```python
from build123d import *

# Parameters (mm, degrees)
SKETCH1_R           = 19.25
SKETCH1_R_2         = 4
BOSS_EXTRUDE1_DEPTH = 4
SKETCH1_4_R         = 4
BOSS_EXTRUDE2_DEPTH = 27.15
CUT_EXTRUDE1_START  = -1.932
SKETCH6_R           = 4
SKETCH6_R_2         = 3.356
CUT_EXTRUDE1_DEPTH  = 1.932
SKETCH7_R           = 2.25
CUT_EXTRUDE2_DEPTH  = 36.735801376
SKETCH8_R           = 2.5
CUT_EXTRUDE3_DEPTH  = 5
CHAMFER1_SIZE       = 2
CHAMFER1_SIZE2      = 0.727940469
SKETCH9_W           = 0.25
SKETCH9_H           = 2.75
CHAMFER3_SIZE       = 0.3
CHAMFER3_SIZE_2     = 0.210062261


with BuildPart() as part:
    # Sketch1 → Boss-Extrude1 (new body)
    # profile 1 of 2: a face of its own
    with BuildSketch(Plane(origin=(0, 0, 0), x_dir=(1, 0, 0), z_dir=(0, 1, 0))):
        with Locations(Location((0, 0, 0), (0, 0, 270))):
            Circle(SKETCH1_R)
        with BuildLine():
            ThreePointArc((2, -16.5), (0, -18.5), (-2, -16.5))
            Line((-2, -16.5), (-2, -16.378339354))
            ThreePointArc((-2, -16.378339354), (-14.289419162, -8.25), (-15.184057953, 6.45711887))
            Line((-15.184057953, 6.45711887), (-15.289419162, 6.517949192))
            ThreePointArc((-15.289419162, 6.517949192), (-16.02146997, 9.25), (-13.289419162, 9.982050808))
            Line((-13.289419162, 9.982050808), (-13.184057953, 9.921220485))
            ThreePointArc((-13.184057953, 9.921220485), (0, 16.5), (13.184057953, 9.921220485))
            Line((13.184057953, 9.921220485), (13.289419162, 9.982050808))
            ThreePointArc((13.289419162, 9.982050808), (16.02146997, 9.25), (15.289419162, 6.517949192))
            Line((15.289419162, 6.517949192), (15.184057953, 6.45711887))
            ThreePointArc((15.184057953, 6.45711887), (16.167667677, 3.294923655), (16.5, 0))
            ThreePointArc((16.5, 0), (12.354149101, -10.937321427), (2, -16.378339354))
            Line((2, -16.378339354), (2, -16.5))
        make_face(mode=Mode.SUBTRACT)
    # profile 2 of 2: a face of its own
    with BuildSketch(Plane(origin=(0, 0, 0), x_dir=(1, 0, 0), z_dir=(0, 1, 0))):
        with BuildLine():
            ThreePointArc((-15.184057953, 6.45711887), (-14.289419162, -8.25), (-2, -16.378339354))
            Line((-2, -16.378339354), (-2, -13.96))
            ThreePointArc((-2, -13.96), (0, -11.96), (2, -13.96))
            Line((2, -13.96), (2, -16.378339354))
            ThreePointArc((2, -16.378339354), (12.354149101, -10.937321427), (16.5, 0))
            ThreePointArc((16.5, 0), (16.167667677, 3.294923655), (15.184057953, 6.45711887))
            Line((15.184057953, 6.45711887), (13.089714637, 5.247949192))
            ThreePointArc((13.089714637, 5.247949192), (10.357663829, 5.98), (11.089714637, 8.712050808))
            Line((11.089714637, 8.712050808), (13.184057953, 9.921220485))
            ThreePointArc((13.184057953, 9.921220485), (0, 16.5), (-13.184057953, 9.921220485))
            Line((-13.184057953, 9.921220485), (-11.094979939, 8.715090731))
            Line((-11.094979939, 8.715090731), (-11.089714637, 8.712050808))
            ThreePointArc((-11.089714637, 8.712050808), (-10.357663829, 5.98), (-13.089714637, 5.247949192))
            Line((-13.089714637, 5.247949192), (-15.184057953, 6.45711887))
        make_face()
        with Locations(Location((0, 0, 0), (0, 0, 270))):
            Circle(SKETCH1_R_2, mode=Mode.SUBTRACT)
    extrude(amount=-BOSS_EXTRUDE1_DEPTH)

    # Sketch1<4> → Boss-Extrude2 (add)
    with BuildSketch(Plane(origin=(0, 0, 0), x_dir=(1, 0, 0), z_dir=(0, 1, 0))):
        with Locations(Location((0, 0, 0), (0, 0, 270))):
            Circle(SKETCH1_4_R)
    extrude(amount=-BOSS_EXTRUDE2_DEPTH)

    # Sketch2 → Cut-Revolve4 (revolve, cut)
    with BuildSketch(Plane(origin=(0, 0, 0), x_dir=(0, 0, -1), z_dir=(1, 0, 0)), mode=Mode.PRIVATE) as cut_revolve4_sk:
        Polygon((0, -27.15), (0.8, -27.15), (0.8, -25.15), (1, 0), (0, 0), align=None)
    revolve(cut_revolve4_sk.sketch.rotate(Axis((0, 0, 0), (0, -1, 0)), 180), axis=Axis((0, 0, 0), (0, -1, 0)), mode=Mode.SUBTRACT)

    # Sketch5 → Cut-Revolve8 (revolve, cut)
    with BuildSketch(Plane.XY, mode=Mode.PRIVATE) as cut_revolve8_sk:
        Polygon((0, -7), (-2.55, -5.527756814), (-2.55, 0), (0, 0), align=None)
    revolve(cut_revolve8_sk.sketch.rotate(Axis((0, 0, 0), (0, -1, 0)), 270), axis=Axis((0, 0, 0), (0, -1, 0)), mode=Mode.SUBTRACT)

    # Sketch6 → Cut-Extrude1 (cut)
    with BuildSketch(Plane.XZ.offset(27.15).offset(CUT_EXTRUDE1_START)):
        with Locations(Location((0, 0, 0), (0, 0, 90))):
            Circle(SKETCH6_R)
        with Locations(Location((0, 0, 0), (0, 0, 270))):
            Circle(SKETCH6_R_2, mode=Mode.SUBTRACT)
    extrude(amount=CUT_EXTRUDE1_DEPTH, mode=Mode.SUBTRACT)

    # Sketch7 → Cut-Extrude2 (cut, through all)
    with BuildSketch(Plane.XZ.offset(4)):
        with Locations(Location((0, -6.25, 0), (0, 0, 270))):
            Circle(SKETCH7_R)
    extrude(amount=-CUT_EXTRUDE2_DEPTH, mode=Mode.SUBTRACT)

    # Sketch8 → Cut-Extrude3 (cut)
    with BuildSketch(Plane(origin=(0, -23, 0), x_dir=(1, 0, 0), z_dir=(0, 1, 0))):
        with Locations((0, 4)):
            Circle(SKETCH8_R)
    extrude(amount=CUT_EXTRUDE3_DEPTH, mode=Mode.SUBTRACT)

    # Chamfer1
    chamfer1_edges = [part.edges().sort_by_distance(p)[0] for p in [
        (0, -18, -4),
    ]]
    chamfer1_side = [part.faces().sort_by_distance(p)[0] for p in [
        (0, -14.609, -4),
    ]]
    chamfer(chamfer1_edges, length=CHAMFER1_SIZE, length2=CHAMFER1_SIZE2, reference=chamfer1_side[0])

    # Sketch9 → Cut-Revolve9 (revolve, cut)
    with BuildSketch(Plane(origin=(0, 0, 0), x_dir=(0, 0, -1), z_dir=(1, 0, 0)), mode=Mode.PRIVATE) as cut_revolve9_sk:
        with Locations((-3.875, -20.5)):
            Rectangle(SKETCH9_W, SKETCH9_H)
    revolve(cut_revolve9_sk.sketch.rotate(Axis((0, -27.15, 0), (0, 1, 0)), 143.580086271), axis=Axis((0, -27.15, 0), (0, 1, 0)), mode=Mode.SUBTRACT)

    # Chamfer3
    # the kernel refuses this chamfer: 0.3, 0.210062261 mm, written as the material it takes off along each edge
    with BuildSketch(Plane(origin=(0, -21.875, 0), x_dir=(-0.42752924874280274, 0, -0.9040015162981834), z_dir=(0.9040015162981834, 0, -0.42752924874280274))) as chamfer3_piece_1_section:
        Polygon((4 - CHAMFER3_SIZE, 0), (4, -CHAMFER3_SIZE_2 * 1.0000000022), (4, 0), align=None)
    chamfer3_piece_1 = revolve(axis=Axis((0, -21.875, 0), (0, 1, 0)), revolution_arc=154.689138052, mode=Mode.PRIVATE)
    chamfer3_piece_1 = chamfer3_piece_1 - Plane(origin=(0, -21.995167344, 0), x_dir=(0.593698599754949, 0, -0.8046874999955033), z_dir=(0, -1, 0)) * Cylinder(3.75, 16, mode=Mode.PRIVATE)
    add(chamfer3_piece_1, mode=Mode.SUBTRACT)
    with BuildSketch(Plane(origin=(0, -21.875, 0), x_dir=(0, 0, 1), z_dir=(-1, 0, 0))) as chamfer3_piece_2_section:
        Polygon((4 - CHAMFER3_SIZE, 0), (4, -CHAMFER3_SIZE_2 * 1.0000000022), (4, 0), align=None)
    chamfer3_piece_2 = revolve(axis=Axis((0, -21.875, 0), (0, 1, 0)), revolution_arc=154.689138052, mode=Mode.PRIVATE)
    chamfer3_piece_2 = chamfer3_piece_2 - Plane(origin=(0, -21.995167344, 0), x_dir=(0.593698599754949, 0, -0.8046874999955033), z_dir=(0, -1, 0)) * Cylinder(3.75, 16, mode=Mode.PRIVATE)
    add(chamfer3_piece_2, mode=Mode.SUBTRACT)


solid = part.part
```
The model under review builds one solid part; all positions refer to its coordinate system, in mm. A direction names the side the tool comes from. Round coordinates to 2 decimals unless told otherwise and drop trailing zeros. Order: outer loops, then holes, each group sorted by start corner. A loop starts at its lowest first (then second) coordinate and runs counter-clockwise, first axis right, second up.
(1) Take a section at C-C, the plane z = 8.5. State the section outline as (x, y) points, plus the area to 3 significant figures.
Working result:
outline: (-17.27, -4) - (17.27, -4) - (17.27, 0) - (-17.27, 0) - close
area: 138 mm2
(2) Take a section at B-B, the plane y = -10.25. State the section outline as (x, z) points, plus the area to 3 significant figures.
Working result:
outline: circle Ø8 at (0, 0); hole circle Ø1.84 at (0, 0)
area: 47.6 mm2
(3) Take a section at D-D, the plane x = -7. State the section outline as (y, z) points, plus the area to 3 significant figures.
Working result:
outline: (-4, -17.93) - (0, -17.93) - (0, 17.93) - (-4, 17.93) - close
area: 143 mm2
(4) Tool access review of faces 4 (the face through (0, -18, -2)), 5 (the face through (-1.532, -23.63, 3.695)), 6 (the face through (-2, -2, 15)), 7 (the face through (-0.77, -2.73, 2.43)): name each direction out of +Z, -Z, +X, -X, +Y, -Y from which nothing blocks a thin tool from reaching the whole face with its end or side.
Working result:
face 4: -Z
face 5: -Y
face 6: +Y, -Y
face 7: +Y
(5) Take a section at A-A, the plane y = -2. State the section outline as (x, z) points.
Working result:
outline: circle Ø38.5 at (0, 0); hole (-15.29, -6.52) arc R2 ccw to (-13.29, -9.98) - (-11.09, -8.71) arc R2 ccw to (-13.09, -5.25) - close; hole circle Ø5.1 at (0, 0); hole circle Ø4.5 at (0, -6.25); hole (-2, 13.96) arc R2 ccw to (2, 13.96) - (2, 16.5) arc R2 ccw to (-2, 16.5) - close; hole (11.09, -8.71) - (13.29, -9.98) arc R2 ccw to (15.29, -6.52) - (13.09, -5.25) arc R2 ccw to start
(6) For P1, Ø5, axis at x = -8, z = 6, coming from the +Y side; P2, Ø1.5, axis at y = -16, z = 4, coming from the -X side; P3, Ø3, axis at x = 0, z = 0, coming from the +Y side; P4, Ø5, axis at x = -3, z = -5.5, coming from the -Y side, all flat-tipped, find the tip position at first contact; note any pin that passes through.
Working result:
P1: stops at y = 0
P2: stops at x = -2.33
P3: stops at y = -6.13
P4: stops at y = -25.22
(7) Mouldability with a two-part tool opening along X and no side actions: class faces 1 (the face through (-18.792, -1.972, -4.173)), 2 (the face through (0, -23, -3)), 3 (the face through (-1, -27.15, 1)) as released by +X, released by -X, zero draft, split by the parting line, or undercut.
Working result:
face 1: split by the parting line
face 2: undercut
face 3: zero draft
(8) Wall thickness on L1, parallel to X at y = -26.7, z = 0; L2, parallel to X at y = -2.9, z = 0; L3, parallel to X at y = -1.2, z = -6.25: over which ranges is each line inside the solid? List them lowest first.
Working result:
L1: x = -3.36 to -0.8, 0.8 to 3.36
L2: x = -19.25 to -2.55, 2.55 to 19.25
L3: x = -18.21 to -14.83, -10.23 to -2.25, 2.25 to 10.23, 14.83 to 18.21
